Autodesk Inventor part; units mm, degrees
ref_plane "YZ Plane" through (0, 0, 0) normal (1, 0, 0) x (0, 1, 0)
ref_plane "XZ Plane" through (0, 0, 0) normal (0, 1, 0) x (-1, 0, 0)
ref_plane "XY Plane" through (0, 0, 0) normal (0, 0, 1) x (1, 0, 0)
sketch "Esboço1" plane through (0, 0, 0) normal (0, 1, 0) x (-1, 0, 0)
  line L0 (0, 0) -> (440, 0)
  line L1 (440, 0) -> (440, -440)
  line L2 (440, -440) -> (0, -440)
  line L3 (0, -440) -> (0, 0)
  dimension "d0" = 440
  dimension "d1" = 440
extrude "Extrusão1" add sketch "Esboço1" along normal blind 2
sketch "Esboço2" plane through (0, 2, 0) normal (0, 1, 0) x (1, 0, 0)
  point P0 (0, 0)
  point P1 (-40, 5)
  point P2 (-47, 5)
  point P3 (-400, 5)
  point P4 (-393, 5)
hole "Furo1" at (-40, 2, -5) at (-47, 2, -5) at (-400, 2, -5) at (-393, 2, -5) direction (0, -1, 0) diameter 2 end through all
fillet "Arredondamento1" radius 2 4 edges at (0, 1, -440) (-440, 1, -440) (-440, 1, 0) (0, 1, 0)
sketch "Esboço3" plane through (0, 2, 0) normal (0, 1, 0) x (1, 0, 0)
  point P0 (0, 0)
  point P1 (-220, 400)
hole "Furo2" at (-220, 2, -400) direction (0, -1, 0) diameter 30 end through all
sketch "Esboço4" plane through (0, 2, 0) normal (0, 1, 0) x (1, 0, 0)
  line L0 (-438, 0) -> (-2, 0)
  line L1 (-34.0574, 0) -> (-52.0574, 0)
  line L2 (-52.0574, 0) -> (-52.0574, 3)
  line L3 (-52.0574, 3) -> (-34.0574, 3)
  line L4 (-34.0574, 3) -> (-34.0574, 0)
  line L5 (-387.0061, 0) -> (-405.0061, 0)
  line L6 (-405.0061, 0) -> (-405.0061, 3)
  line L7 (-405.0061, 3) -> (-387.0061, 3)
  line L8 (-387.0061, 3) -> (-387.0061, 0)
  point P0 (0, 0)
  dimension "d19" = 18
  dimension "d20" = 3
  dimension "d21" = 18
  dimension "d22" = 3
extrude "Extrusão2" cut sketch "Esboço4" against normal blind 2
properties part number "porta" material "Acrílico"
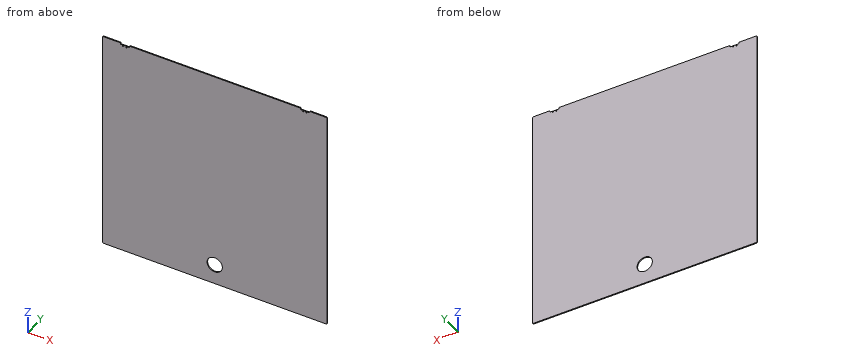
Source: CAD feature listing. Evaluate the final solid. Frame: model axes, mm. Coordinates: 2 decimals unless noted, no trailing zeros. Loops run counter-clockwise (first coordinate to the right, second up) from the corner with the lowest first, then second, coordinate; pieces in that order, holes last. Notation, with made-up numbers: (18, 22.25) - (48, 22.25) arc R16 ccw to (48, 38.25) - close; hole circle Ø2 at (-5.75, 44). An arc over 180 degrees is marked (long way). Answer as CSV lines item,"result".
1. Section A-A (z = -400). Return loops of the section in (x, y).
Established:
outline,"(-440, 0) - (-235, 0) - (-235, 2) - (-440, 2) - close; (-205, 0) - (0, 0) - (0, 2) - (-205, 2) - close"
2. Section B-B (x = -220). Return loops of the section in (y, z).
Established:
outline,"(0, -440) - (2, -440) - (2, -415) - (0, -415) - close; (0, -385) - (2, -385) - (2, 0) - (0, 0) - close"
3. Contact query for flat-ended pins moving along their axis: pin 1 (1 mm diameter, centred on x = -399, y = 1.5, fed in from +Z); pin 2 (0.6 mm diameter, centred on y = 1, z = -1.5, fed in from +X). Output: stop coordinate, or through.
Established:
pin 1,"stops at z = -3"
pin 2,"stops at x = -0.01"
4. Ray query, line 1 (X direction, y = 0.7, z = -5); line 2 (Z direction, x = -393, y = 1.6); line 3 (Z direction, x = -403, y = 1.65). Return the intervals inside material, ascending.
Established:
line 1,"x = -440 to -401, -399 to -394, -392 to -48, -46 to -41, -39 to 0"
line 2,"z = -440 to -6, -4 to -3"
line 3,"z = -440 to -3"
